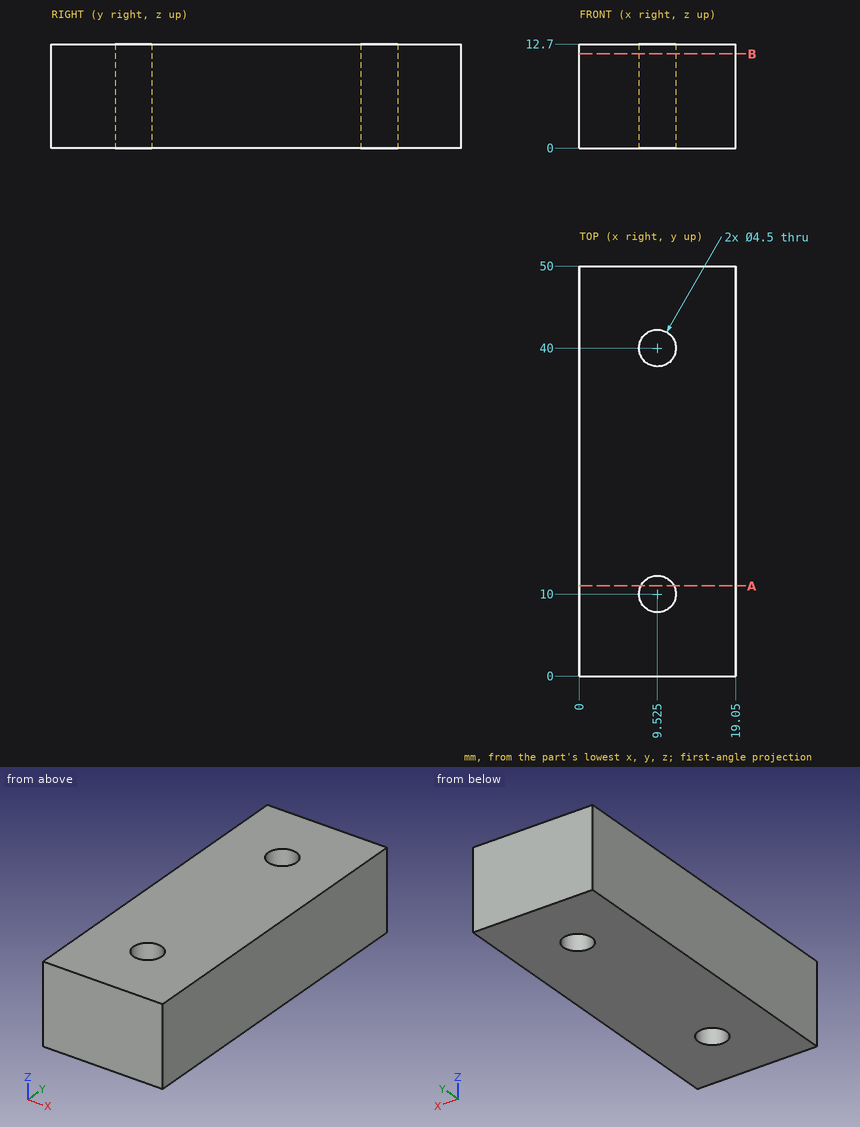
Geometry: see drawing. Coordinates: mm, zero at the bounding-box minimum. Round coordinates to 2 decimals unless told otherwise and drop trailing zeros. Order: outer loops, then holes, each group sorted by start corner. A loop starts at its lowest first (then second) coordinate and runs counter-clockwise, first axis right, second up. Notation, with made-up numbers: (10, 71.25) - (31, 71.25) arc R23 ccw to (31, 96.25) - close; hole circle Ø7 at (28.25, -10.75). An arc over 180 degrees is marked (long way). Use a Markdown table: item, result. Add a question column.
1. Section query A-A (y = 11). Return the cut outline in (x, z), then the cut area to 3 significant figures.
2. Line query: probe 1 along Y at (x, z) = (9.75, 6); probe 2 along Y at (x, z) = (10.25, 2); probe 3 along X at (y, z) = (9.5, 11). Output: solid intervals per line, ascending.
3. Section query B-B (z = 11.5). Return the cut outline in (x, y) (3 decimals), then the cut area to 3 significant figures.
4. First-contact query: pin 1 (2 mm diameter, centred on x = 12.5, z = 3, fed in from -Y). Flat tip, straight axial feed; report the tip coordinate or a pass-through.
Derived:
| question | item | result |
|---|---|---|
| 1 | outline | (0, 0) - (7.51, 0) - (7.51, 12.7) - (0, 12.7) - close; (11.54, 0) - (19.05, 0) - (19.05, 12.7) - (11.54, 12.7) - close |
| 1 | area | 191 mm2 |
| 2 | probe 1 | 0 to 7.76, 12.24 to 37.76, 42.24 to 50 |
| 2 | probe 2 | 0 to 7.87, 12.13 to 37.87, 42.13 to 50 |
| 2 | probe 3 | 0 to 7.33, 11.72 to 19.05 |
| 3 | outline | (0, 0) - (19.05, 0) - (19.05, 50) - (0, 50) - close; hole circle Ø4.5 at (9.525, 10); hole circle Ø4.5 at (9.525, 40) |
| 3 | area | 921 mm2 |
| 4 | pin 1 | y = 0 |
